```python
from build123d import *

# Parameters (mm, degrees)
F0_W        = 9.525
F0_H        = 13.4751944874
F0_W_2      = 3.175
F0_H_2      = 15.7348055126
F0_H_3      = 17.78
F0_H_4      = 3.81
F1_DEPTH    = 1.55575
F0_W_3      = 3.81
F0_H_5      = 31.4696110251
F0_W_4      = 6.35
F0_H_6      = 1.27
F0_H_7      = 19.05
F0_H_8      = 2.2596110251
F0_W_5      = 2.2601685487
F2_DEPTH    = 3.175
F3_R        = 1
F4_DEPTH    = 15.84325
F5_SIZE     = 3
F6_T1_DEPTH = 203.7288380727
F8_DEPTH    = 25.4


# Not quite as in the source:
# - a fillet or chamfer that OpenCascade refuses, or shapes differently, is made with other operations: its cross-section is extruded or revolved along the edge and cut away or added


with BuildPart() as f1:
    # F0 (on Top) → F1 (new body)
    with BuildSketch(Plane.XY):
        with Locations((-4.7625, 26.2824027563)):
            Rectangle(F0_W, F0_H)
        with Locations((-11.1125, 26.2824027563)):
            Rectangle(F0_W_2, F0_H)
        with Locations((-11.1125, 11.6774027563)):
            Rectangle(F0_W_2, F0_H_2)
        with Locations((-4.7625, 11.6774027563)):
            Rectangle(F0_W, F0_H_2)
        with Locations((4.7625, 11.6774027563)):
            Rectangle(F0_W, F0_H_2)
        with Locations((11.1125, 11.6774027563)):
            Rectangle(F0_W_2, F0_H_2)
        with Locations((11.1125, 26.2824027563)):
            Rectangle(F0_W_2, F0_H)
        Polygon((0, 33.02), (0, 19.5448055126), (9.525, 19.5448055126), (9.525, 33.02), (2.2601685487, 33.02), align=None)
        with Locations((-4.7625, -8.89)):
            Rectangle(F0_W, F0_H_3)
        with Locations((4.7625, -8.89)):
            Rectangle(F0_W, F0_H_3)
        with Locations((11.1125, -8.89)):
            Rectangle(F0_W_2, F0_H_3)
        with Locations((-11.1125, -8.89)):
            Rectangle(F0_W_2, F0_H_3)
        with Locations((-11.1125, 1.905)):
            Rectangle(F0_W_2, F0_H_4)
        with Locations((-4.7625, 1.905)):
            Rectangle(F0_W, F0_H_4)
        with Locations((4.7625, 1.905)):
            Rectangle(F0_W, F0_H_4)
        with Locations((11.1125, 1.905)):
            Rectangle(F0_W_2, F0_H_4)
    extrude(amount=F1_DEPTH)

    # F0 (on Top) → F2 (join)
    with BuildSketch(Plane.XY):
        Polygon((-12.7, 33.02), (-9.525, 33.02), (-9.525, 35.2796110251), (-19.05, 35.2796110251), (-19.05, 19.5448055126), (-12.7, 19.5448055126), align=None)
        with Locations((-14.2875, 37.1846110251)):
            Rectangle(F0_W, F0_H_4)
        with Locations((-20.955, 37.1846110251)):
            Rectangle(F0_W_3, F0_H_4)
        with Locations((-24.765, 37.1846110251)):
            Rectangle(F0_W_3, F0_H_4)
        with Locations((-24.765, 19.5448055126)):
            Rectangle(F0_W_3, F0_H_5)
        with Locations((-24.765, 1.905)):
            Rectangle(F0_W_3, F0_H_4)
        with Locations((-20.955, 1.905)):
            Rectangle(F0_W_3, F0_H_4)
        with Locations((-15.875, 1.905)):
            Rectangle(F0_W_4, F0_H_4)
        with Locations((-15.875, 11.6774027563)):
            Rectangle(F0_W_4, F0_H_2)
        Polygon((-9.525, -19.05), (-9.525, -17.78), (-12.7, -17.78), (-12.7, 0), (-19.05, 0), (-14.2875, -19.05), align=None)
        with Locations((-4.7625, -18.415)):
            Rectangle(F0_W, F0_H_6)
        with Locations((4.7625, -18.415)):
            Rectangle(F0_W, F0_H_6)
        Polygon((12.7, -17.78), (9.525, -17.78), (9.525, -19.05), (14.2875, -19.05), (19.05, 0), (12.7, 0), align=None)
        Polygon((14.2875, -19.05), (9.525, -19.05), (9.525, -38.1), align=None)
        Polygon((-9.525, -38.1), (-9.525, -19.05), (-14.2875, -19.05), align=None)
        with Locations((-4.7625, -28.575)):
            Rectangle(F0_W, F0_H_7)
        with Locations((4.7625, -28.575)):
            Rectangle(F0_W, F0_H_7)
        with Locations((15.875, 1.905)):
            Rectangle(F0_W_4, F0_H_4)
        with Locations((15.875, 11.6774027563)):
            Rectangle(F0_W_4, F0_H_2)
        Polygon((9.525, 35.2796110251), (9.525, 33.02), (12.7, 33.02), (12.7, 19.5448055126), (19.05, 19.5448055126), (19.05, 35.2796110251), align=None)
        with Locations((-4.7625, 34.1498055126)):
            Rectangle(F0_W, F0_H_8)
        with Locations((-4.7625, 37.1846110251)):
            Rectangle(F0_W, F0_H_4)
        with Locations((1.1300842743, 37.1846110251)):
            Rectangle(F0_W_5, F0_H_4)
        with Locations((14.2875, 37.1846110251)):
            Rectangle(F0_W, F0_H_4)
        with Locations((20.955, 37.1846110251)):
            Rectangle(F0_W_3, F0_H_4)
        with Locations((24.765, 37.1846110251)):
            Rectangle(F0_W_3, F0_H_4)
        with Locations((24.765, 19.5448055126)):
            Rectangle(F0_W_3, F0_H_5)
        with Locations((24.765, 1.905)):
            Rectangle(F0_W_3, F0_H_4)
        with Locations((20.955, 1.905)):
            Rectangle(F0_W_3, F0_H_4)
        with Locations((1.1300842743, 34.1498055126)):
            Rectangle(F0_W_5, F0_H_8)
    extrude(amount=F2_DEPTH)

    # F3
    f3_edges = [f1.edges().sort_by_distance(p)[0] for p in [
        (26.67, 19.544806, 3.175),
        (22.86, 0, 3.175),
        (26.67, 0, 1.5875),
        (26.67, 39.089611, 1.5875),
        (-12.204916, 39.089611, 3.175),
        (18.0975, 39.089611, 3.175),
        (20.955, 35.279611, 3.175),
        (20.955, 3.81, 3.175),
        (22.86, 19.544806, 3.175),
        (-26.67, 19.544806, 3.175),
        (-22.86, 0, 3.175),
        (-26.67, 0, 1.5875),
        (-22.86, 19.544806, 3.175),
        (-20.955, 35.279611, 3.175),
        (-26.67, 39.089611, 1.5875),
        (-20.955, 3.81, 3.175),
    ]]
    fillet(f3_edges, radius=F3_R)

    # F0 (on Top) → F4 (join)
    with BuildSketch(Plane.XY):
        with Locations((-14.2875, 37.1846110251)):
            Rectangle(F0_W, F0_H_4)
        Polygon((-12.7, 33.02), (-9.525, 33.02), (-9.525, 35.2796110251), (-19.05, 35.2796110251), (-19.05, 19.5448055126), (-12.7, 19.5448055126), align=None)
        with Locations((-4.7625, 34.1498055126)):
            Rectangle(F0_W, F0_H_8)
        with Locations((-4.7625, 37.1846110251)):
            Rectangle(F0_W, F0_H_4)
        with Locations((1.1300842743, 37.1846110251)):
            Rectangle(F0_W_5, F0_H_4)
        with Locations((1.1300842743, 34.1498055126)):
            Rectangle(F0_W_5, F0_H_8)
        with Locations((14.2875, 37.1846110251)):
            Rectangle(F0_W, F0_H_4)
        Polygon((9.525, 35.2796110251), (9.525, 33.02), (12.7, 33.02), (12.7, 19.5448055126), (19.05, 19.5448055126), (19.05, 35.2796110251), align=None)
        with Locations((15.875, 11.6774027563)):
            Rectangle(F0_W_4, F0_H_2)
        with Locations((15.875, 1.905)):
            Rectangle(F0_W_4, F0_H_4)
        Polygon((12.7, -17.78), (9.525, -17.78), (9.525, -19.05), (14.2875, -19.05), (19.05, 0), (12.7, 0), align=None)
        with Locations((4.7625, -18.415)):
            Rectangle(F0_W, F0_H_6)
        with Locations((-4.7625, -18.415)):
            Rectangle(F0_W, F0_H_6)
        Polygon((-9.525, -19.05), (-9.525, -17.78), (-12.7, -17.78), (-12.7, 0), (-19.05, 0), (-14.2875, -19.05), align=None)
        with Locations((-15.875, 11.6774027563)):
            Rectangle(F0_W_4, F0_H_2)
        with Locations((-15.875, 1.905)):
            Rectangle(F0_W_4, F0_H_4)
        Polygon((-9.525, -38.1), (-9.525, -19.05), (-14.2875, -19.05), align=None)
        Polygon((14.2875, -19.05), (9.525, -19.05), (9.525, -38.1), align=None)
        with Locations((4.7625, -28.575)):
            Rectangle(F0_W, F0_H_7)
        with Locations((-4.7625, -28.575)):
            Rectangle(F0_W, F0_H_7)
    extrude(amount=F4_DEPTH)

    # F5
    f5_edges = [f1.edges().sort_by_distance(p)[0] for p in [
        (-19.05, 19.544806, 15.84325),
        (-8.394916, 39.089611, 15.84325),
        (14.2875, 39.089611, 15.84325),
        (19.05, 19.544806, 15.84325),
    ]]
    chamfer(f5_edges, length=F5_SIZE)

    # F6: chamfer of 35.56 x 9.5282732829 on 1 edges, made by hand

    # F6_s2 → F6_t1 (cut)
    with BuildSketch(Plane.YZ.offset(-101.8644190363)):
        Polygon((-2.54, 15.84325), (-38.1, 6.3149767171), (-38.1, 15.84325), align=None)
    extrude(amount=F6_T1_DEPTH, mode=Mode.SUBTRACT)

    # F7 (on face) → F8 (cut)
    with BuildSketch(Plane(origin=(9.525, 0, 0), x_dir=(0, -1, 0), z_dir=(-1, 0, 0))):
        with BuildLine():
            ThreePointArc((-34.5021110251, 9.49325), (-34.96707901, 10.6157820151), (-36.0896110251, 11.08075))
            ThreePointArc((-36.0896110251, 11.08075), (-37.2121430402, 8.3707179849), (-34.5021110251, 9.49325))
        make_face()
    extrude(amount=-F8_DEPTH, mode=Mode.SUBTRACT)


solid = f1.part
```
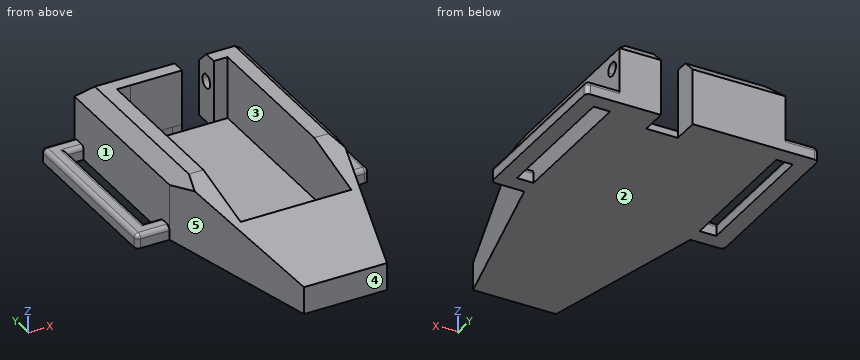
The model under review builds one solid part; all positions refer to its coordinate system, in mm. Face numbers are marked on the shaded views. A direction names the side the tool comes from. Give positions to 0.01 mm unless a question says otherwise; leave off trailing zeros. Loops run counter-clockwise (first coordinate to the right, second up) from the corner with the lowest first, then second, coordinate; pieces in that order, holes last. Notation, with made-up numbers: (3.5, -30.5) -> (31.5, -30.5) arc R12 ccw to (31.5, -19.5) -> close; hole circle Ø11 at (45.25, 14). An arc over 180 degrees is marked (long way). Use CSV: the item, a comma, the result in double quotes.
1. Consider section A-A, the plane y = 9. Write out the cut boundary in (x, z) (3 decimals), then the cut area to 3 significant figures.
Result:
outline,"(-26.67, 0) -> (-22.86, 0) -> (-22.86, 2.175) arc R1 ccw to (-23.86, 3.175) -> (-25.67, 3.175) arc R1 ccw to (-26.67, 2.175) -> close; (-19.05, 0) -> (19.05, 0) -> (19.05, 12.843) -> (16.05, 15.843) -> (12.7, 15.843) -> (12.7, 1.556) -> (-12.7, 1.556) -> (-12.7, 15.843) -> (-16.05, 15.843) -> (-19.05, 12.843) -> close; (22.86, 0) -> (26.67, 0) -> (26.67, 2.175) arc R1 ccw to (25.67, 3.175) -> (23.86, 3.175) arc R1 ccw to (22.86, 2.175) -> close"
area,"255 mm²"
2. To check wall thickness, follow probe 1 along X at (y, z) = (30.5, 11.75); probe 2 along X at (y, z) = (27, 3); probe 3 along Y at (x, z) = (-21, 1.75). State the ranges of each line that lie inside material, in increasing order. Write a range as from..to.
Result:
probe 1,"x = -19.05..-12.7, 12.7..19.05"
probe 2,"x = -26.24..-23.29, -19.05..-12.7, 12.7..19.05, 23.29..26.24"
probe 3,"y = 0..3.81, 35.28..39.09"
3. Consider section D-D, the plane x = 10.5. Write out the cut boundary in (y, z) (1 decimal).
Result:
outline,"(-34.2, 0) -> (39.1, 0) -> (39.1, 12.8) -> (36.1, 15.8) -> (33, 15.8) -> (33, 1.6) -> (-17.8, 1.6) -> (-17.8, 11.8) -> (-34.2, 7.4) -> close; hole circle Ø3.2 at (36.1, 9.5)"
4. Consider section C-C, the plane z = 4.5. Write out the cut boundary in (x, y) (3 decimals).
Result:
outline,"(-19.05, 0) -> (-9.525, -38.1) -> (9.525, -38.1) -> (19.05, 0) -> (19.05, 39.09) -> (9.525, 39.09) -> (9.525, 33.02) -> (12.7, 33.02) -> (12.7, -17.78) -> (-12.7, -17.78) -> (-12.7, 33.02) -> (2.26, 33.02) -> (2.26, 39.09) -> (-19.05, 39.09) -> close"
5. For P1, Ø4, axis at y = -11.5, z = 2, coming from the -X side (3 decimals); P2, Ø6, axis at y = 22, z = 11, coming from the -X side; P3, Ø0.7, axis at x = 22.5, z = 1, coming from the -Y side; P4, Ø4, axis at x = 18.5, y = 11.5, coming from the -Z side, all flat-tipped, find the tip position at first contact; note any pin that passes through.
Result:
P1,"stops at x = -16.675"
P2,"stops at x = -19.05"
P3,"stops at y = 0"
P4,"stops at z = 0"
6. Machinability: for the marked faces 1 and 2, which of the approach directions +Z, -Z, +X, -X, +Y, -Y give a long, thin tool a straight path to every point of the face, cutting with its end or side? Answer none if there is none.
Result:
face 1,"+Z"
face 2,"-Z, +X, -X, +Y, -Y"
7. Consider section B-B, the plane x = -8. Write out the cut boundary in (y, z), then the cut area to 3 significant figures.
Result:
outline,"(-38.1, 0) -> (39.09, 0) -> (39.09, 12.84) -> (36.09, 15.84) -> (33.02, 15.84) -> (33.02, 1.56) -> (-17.78, 1.56) -> (-17.78, 11.76) -> (-38.1, 6.31) -> close"
area,"354 mm²"
8. The part is to be moulded in two halves that separate along X. For the marked faces 3, 4 and 5, say which applies: +X half, -X half, draft (parallel to the pull), parting line (faces both ways), or undercut.
Result:
face 3,"undercut"
face 4,"draft"
face 5,"-X half"
